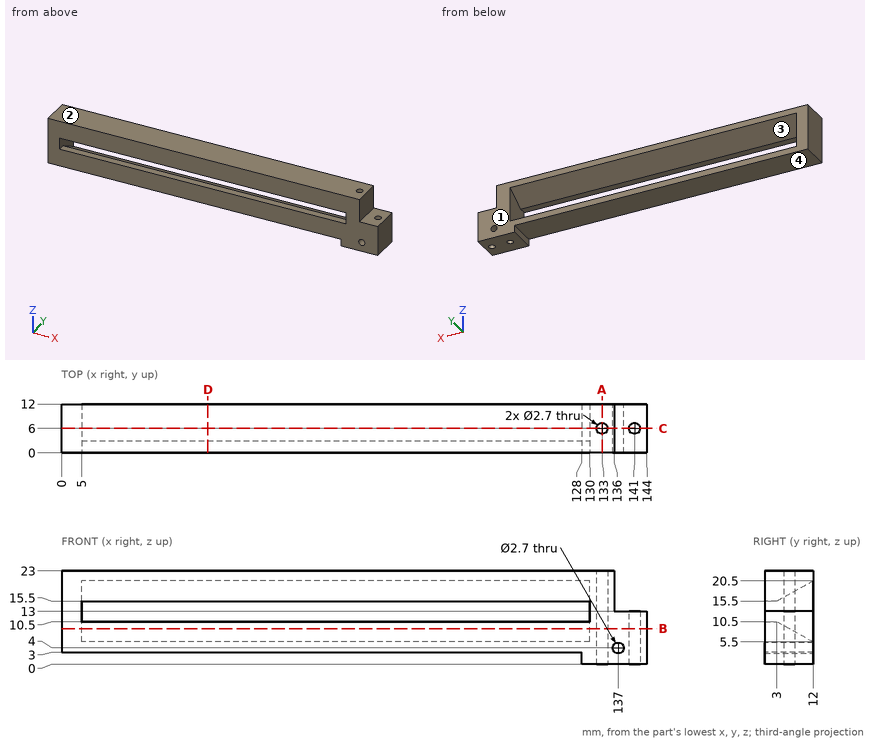
For this review, use the dimensioned drawing (mm, ordinates from the lowest corner) and the shaded views. Round coordinates to 2 decimals unless told otherwise and drop trailing zeros. Loops run counter-clockwise (first coordinate to the right, second up) from the corner with the lowest first, then second, coordinate; pieces in that order, holes last. Notation, with made-up numbers: M -31,60 L -5,60 A25 cw -5,96 Z; hole C 66.5,58 d2. An arc over 180 degrees is marked long. Answer as a JSON object with one key per item and string values.
(1) Clearance check with flat-ended pins moving along their axes: P1, Ø3, axis at x = 95.5, z = 11.5, coming from the +Y side; P2, Ø4, axis at x = 139, y = 4.5, coming from the +Z side; P3, Ø3.5, axis at x = 51, y = 7.5, coming from the -Z side. State where each tip first meets the part, or that it passes through.
Resolved:
{"P1": "y = 3.9", "P2": "z = 13", "P3": "z = 3"}
(2) Take a section at B-B on z = 8.75. Give the boundary of the cut face in (x, y).
Resolved:
{"outline": "M 0,0 L 144,0 L 144,12 L 130,12 L 130,6.15 L 5,6.15 L 5,12 L 0,12 Z; hole C 133,6 d2.7; hole C 141,6 d2.7"}
(3) Draft analysis for pull direction Z (two halves, no side actions). For the marked faces 1, 2, 3 and 4, state which applies: released by +Z, released by -Z, zero draft, split by the parting line, or undercut.
Resolved:
{"face 1": "zero draft", "face 2": "released by +Z", "face 3": "undercut", "face 4": "released by -Z"}
(4) Take a section at C-C on y = 6. Give the boundary of the cut face in (x, z), and give its area (3 significant figures).
Resolved:
{"outline": "M 0,3 L 128,3 L 128,0 L 131.65,0 L 131.65,23 L 0,23 Z; M 134.35,0 L 139.65,0 L 139.65,13 L 136,13 L 136,23 L 134.35,23 Z; M 142.35,0 L 144,0 L 144,13 L 142.35,13 Z; hole M 5,8.83 L 130,8.83 L 130,17.17 L 5,17.17 Z; hole C 137,4 d2.7", "area": "1,700 mm²"}
(5) To check wall thickness, follow line 1 along X through (y, z) = (6.25, 1.25); line 2 along Z through (x, y) = (83.5, 2.5); line 3 along X through (y, z) = (0.75, 12). State the ranges of each line that lie inside material, in increasing order.
Resolved:
{"line 1": "128 to 131.67, 134.33 to 139.67, 142.33 to 144", "line 2": "3 to 10.5, 15.5 to 23", "line 3": "0 to 5, 130 to 144"}
(6) Take a section at D-D on x = 36. Give the boundary of the cut face in (y, z).
Resolved:
{"outline": "M 0,3 L 12,3 L 12,5.5 L 3,10.5 L 0,10.5 Z; M 0,15.5 L 3,15.5 L 12,20.5 L 12,23 L 0,23 Z"}
(7) Take a section at A-A on x = 133. Give the boundary of the cut face in (y, z).
Resolved:
{"outline": "M 0,0 L 4.65,0 L 4.65,23 L 0,23 Z; M 7.35,0 L 12,0 L 12,23 L 7.35,23 Z"}
